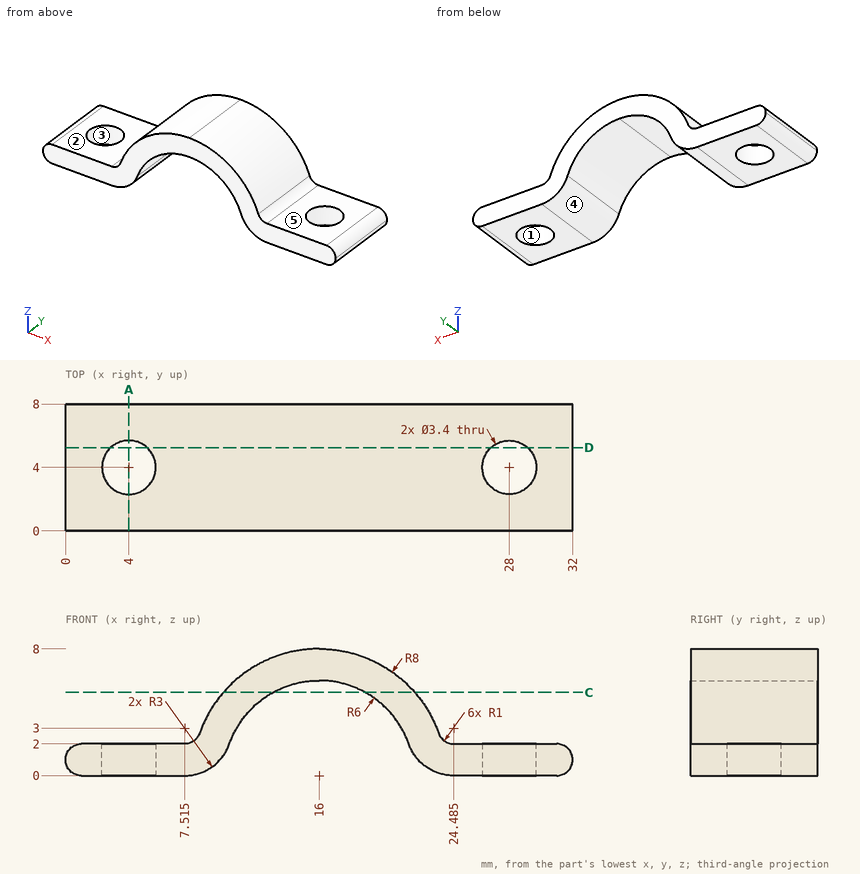
The figure shows three views and two pictorial views of one solid part (mm, origin at its lowest corner). Answer the questions. A direction names the side the tool comes from. Coordinates: 2 decimals unless noted, no trailing zeros. Write each loop counter-clockwise with the first axis right and the second up, starting at its lowest first coordinate (ties: lowest second). Pieces come first, ordered by that corner, then holes. Notation, with made-up numbers: (88.5, 40) -> (141.5, 40) arc R24 ccw to (141.5, 56) -> close; hole circle Ø4 at (-34.75, 55). An arc over 180 degrees is marked (long way). Return JSON: item names as keys, results as strings.
1. Determine the mould class of the marked faces 1 and 2 for opening direction X: pulls with the +X half, pulls with the -X half, needs draft (parallel to the pull), parting line crosses it, or undercut.
Found:
{"face 1": "undercut", "face 2": "needs draft"}
2. A tool of negligible diameter and unlimited length cuts with its end or side. For the marked faces 3, 4 and 5, from which of +Z, -Z, +X, -X, +Y, -Y can it reach the whole face along a straight path? Write none if from no direction.
Found:
{"face 3": "+Z, -Z", "face 4": "-Z, +Y, -Y", "face 5": "+Z, +X, +Y, -Y"}
3. Find the intervals of material crossed by line 1 along Y through (x, z) = (28, 1.5); line 2 along Z through (x, y) = (29.5, 6.75); line 3 along Y through (x, z) = (26.5, 1.25), in increasing order. Write a range as from..to.
Found:
{"line 1": "0..2.3, 5.7..8", "line 2": "0..2", "line 3": "0..3.2, 4.8..8"}
4. This flat-tipped pin is pushed along its axis until it touches: P1, Ø3, axis at x = 27.5, y = 2.5, coming from the -Z side. Where does it stop, or does it pass through?
Found:
{"P1": "z = 0"}
5. A cutting plane is placed at C-C (z = 5.25). Determine the outline of the cut face in (x, y) (1 decimal), and give its area (3 significant figures).
Found:
{"outline": "(10, 0) -> (13.1, 0) -> (13.1, 8) -> (10, 8) -> close; (18.9, 0) -> (22, 0) -> (22, 8) -> (18.9, 8) -> close", "area": "50.1 mm2"}
6. A cutting plane is placed at A-A (x = 4). Determine the outline of the cut face in (y, z).
Found:
{"outline": "(0, 0) -> (2.3, 0) -> (2.3, 2) -> (0, 2) -> close; (5.7, 0) -> (8, 0) -> (8, 2) -> (5.7, 2) -> close"}
7. A cutting plane is placed at D-D (y = 5.25). Give the number of separate pieces and of enclosed holes in the cut face, and give its area (3 significant figures).
Found:
{"separate pieces": "3", "enclosed holes": "0", "area": "64.3 mm2"}
